Read the model definition and answer for the solid it produces. Units are mm, in the model's axes. Give positions to 0.01 mm unless a question says otherwise; leave off trailing zeros. Order: outer loops, then holes, each group sorted by start corner. A loop starts at its lowest first (then second) coordinate and runs counter-clockwise, first axis right, second up. Notation, with made-up numbers: (1.5, 15.5) - (29.5, 15.5) arc R21 ccw to (29.5, 39.5) - close; hole circle Ø2 at (0.25, -15.5). An arc over 180 degrees is marked (long way). One line per item, written item: value. Start each with the question number.
```python
from build123d import *

# Parameters (mm, degrees)
SKETCH1_W            = 147.29
SKETCH1_H            = 100
BOSS_EXTRUDE1_DEPTH  = 3
M3_CLEARANCE_HOLE2_D = 3.4
M3_CLEARANCE_HOLE3_D = 3.4
FILLET1_R            = 5


with BuildPart() as part:
    # Sketch1 → Boss-Extrude1 (new body)
    with BuildSketch(Plane(origin=(0, 0, 0), x_dir=(0, 0, -1), z_dir=(1, 0, 0))):
        Rectangle(SKETCH1_W, SKETCH1_H)
    extrude(amount=BOSS_EXTRUDE1_DEPTH)

    # M3 Clearance Hole2 (through all)
    with Locations(Plane(origin=(3, 0, 0), x_dir=(0, 0, -1), z_dir=(1, 0, 0))):
        with Locations((58.645, -35), (51.645, -35), (58.645, -28), (65.645, -35), (58.645, -42), (58.645, 35), (58.645, 42), (51.645, 35), (58.645, 28), (65.645, 35)):
            Hole(M3_CLEARANCE_HOLE2_D / 2)

    # M3 Clearance Hole3 (through all)
    with Locations(Plane.ZY):
        with Locations((58.645, 35), (58.645, 42), (65.645, 35), (58.645, 28), (51.645, 35), (58.645, -35), (58.645, -28), (65.645, -35), (58.645, -42), (51.645, -35)):
            Hole(M3_CLEARANCE_HOLE3_D / 2)

    # Fillet1
    fillet1_edges = [part.edges().sort_by_distance(p)[0] for p in [
        (1.5, -50, -73.645),
        (1.5, -50, 73.645),
        (1.5, 50, 73.645),
        (1.5, 50, -73.645),
    ]]
    fillet(fillet1_edges, radius=FILLET1_R)


solid = part.part
```
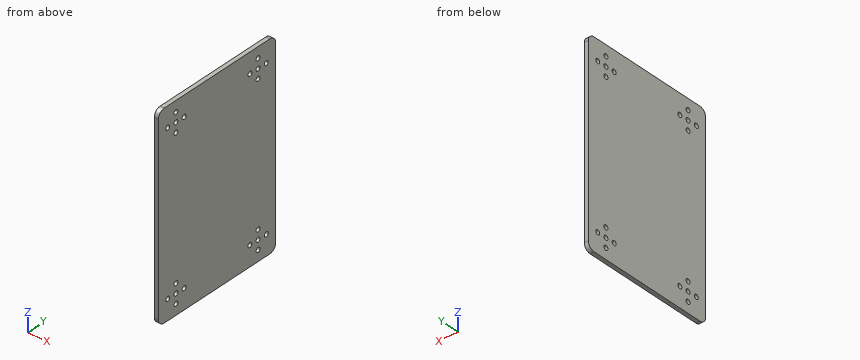
1) Section A-A on y = -42 is taken. Write down the section's boundary in (x, z) (3 decimals), plus the area to 3 significant figures.
2) This flat-tipped pin is pushed along its axis until it touches: pin 1 (2 mm diameter, centred on y = 28, z = -58.645, fed in from +X). Where does it stop, or does it pass through?
3) Find the intervals of material crossed by probe 1 along Y at (x, z) = (0.2, -51.5); probe 2 along Z at (x, y) = (0.5, -29.5) (3 decimals); probe 3 along Z at (x, y) = (1.35, -41) (3 decimals), in increasing order. Write a range as from..to.
Solved:
1. outline: (0, -73.645) - (3, -73.645) - (3, -60.345) - (0, -60.345) - close; (0, -56.945) - (3, -56.945) - (3, 56.945) - (0, 56.945) - close; (0, 60.345) - (3, 60.345) - (3, 73.645) - (0, 73.645) - close
1. area: 421 mm2
2. pin 1: passes through
3. probe 1: y = -50..-36.69, -33.31..33.31, 36.69..50
3. probe 2: z = -73.645..-59.445, -57.845..57.845, 59.445..73.645
3. probe 3: z = -73.645..-60.02, -57.27..57.27, 60.02..73.645
